```python
from build123d import *

# Parameters (mm, degrees)
SALIENTE_EXTRUIR1_DEPTH = 25.2


with BuildPart() as part:
    # Croquis1 → Saliente-Extruir1 (new body)
    with BuildSketch(Plane(origin=(0, 0, 0), x_dir=(1, 0, 0), z_dir=(0, 1, 0))):
        with BuildLine():
            Line((-2.5, 11.55), (2.5, 11.55))
            Line((2.5, 11.55), (2.5, 9.16515139))
            ThreePointArc((2.5, 9.16515139), (0, -9.5), (-2.5, 9.16515139))
            Line((-2.5, 9.16515139), (-2.5, 11.55))
        make_face()
        with BuildLine():
            Line((-2.439487651, 3.17), (2.439487651, 3.17))
            ThreePointArc((2.439487651, 3.17), (0, -4), (-2.439487651, 3.17))
        make_face(mode=Mode.SUBTRACT)
    extrude(amount=SALIENTE_EXTRUIR1_DEPTH)


solid = part.part
```
Check sheet for the modelled part. Datum: model origin and axes. Units: mm. A direction names the side the tool comes from. Give positions to 0.01 mm unless a question says otherwise; leave off trailing zeros. Order: outer loops, then holes, each group sorted by start corner. A loop starts at its lowest first (then second) coordinate and runs counter-clockwise, first axis right, second up. Notation, with made-up numbers: (43, 49.5) -> (90, 49.5) arc R15 ccw to (90, 65.5) -> close; hole circle Ø3 at (-13.5, 63). An arc over 180 degrees is marked (long way). Return JSON: item names as keys, results as strings.
1. Cross-section at A-A, the plane x = 0. Record the cut outline in (y, z).
From the geometry:
{"outline": "(0, -11.55) -> (25.2, -11.55) -> (25.2, -3.17) -> (0, -3.17) -> close; (0, 4) -> (25.2, 4) -> (25.2, 9.5) -> (0, 9.5) -> close"}
2. Mould release check, pull along X, two halves, no side actions. Record for faces 4 (the flat face through (2.5, 12, -10)), 5 (the cylindrical face through (0, 12, 4)), 6 (the cylindrical face through (0.382, 12.424, 9.492)): +X half, -X half, draft (parallel to the pull), parting line (faces both ways), or undercut.
From the geometry:
{"face 4": "+X half", "face 5": "undercut", "face 6": "parting line"}
3. Cross-section at C-C, the plane y = 13.75. Record the cut outline in (x, z).
From the geometry:
{"outline": "(-2.5, -11.55) -> (2.5, -11.55) -> (2.5, -9.17) arc R9.5 ccw (long way) to (-2.5, -9.17) -> close; hole (-2.44, -3.17) -> (2.44, -3.17) arc R4 ccw (long way) to start"}
4. Set-up check for faces 1 (the flat face through (0, 12, -3.17)), 2 (the flat face through (-2.5, 12, -10)), 3 (the flat face through (0, 12, -11.55)): record each of +Z, -Z, +X, -X, +Y, -Y from which the full face is reachable in a straight line by a thin tool's end or side.
From the geometry:
{"face 1": "+Y, -Y", "face 2": "-Z, -X, +Y, -Y", "face 3": "-Z, +X, -X, +Y, -Y"}
5. Material ranges on probe 1 along X at (y, z) = (12, 0); probe 2 along Z at (x, y) = (0.25, 9.25); probe 3 along Z at (x, y) = (-1.25, 5.75), recorded low to high. Write a range as [from, to].
From the geometry:
{"probe 1": "[-9.5, -4], [4, 9.5]", "probe 2": "[-11.55, -3.17], [3.99, 9.5]", "probe 3": "[-11.55, -3.17], [3.8, 9.42]"}
6. Cross-section at D-D, the plane z = 5.5. Record the cut outline in (x, y), plus the area to 3 significant figures.
From the geometry:
{"outline": "(-7.75, 0) -> (7.75, 0) -> (7.75, 25.2) -> (-7.75, 25.2) -> close", "area": "390 mm^2"}
7. Go/stop test with flat-tipped pins: P1, Ø1, axis at y = 5, z = 5, coming from the -X side; P2, Ø10, axis at y = 20, z = 7, coming from the +X side; P3, Ø4, axis at y = 6.5, z = -6.5, coming from the +X side. Record where each tip stops, or that it passes through.
From the geometry:
{"P1": "x = -8.37", "P2": "x = 9.29", "P3": "x = 8.37"}
8. Cross-section at B-B, the plane z = 0. Record the cut outline in (x, y), plus the area to 3 significant figures.
From the geometry:
{"outline": "(-9.5, 0) -> (-4, 0) -> (-4, 25.2) -> (-9.5, 25.2) -> close; (4, 0) -> (9.5, 0) -> (9.5, 25.2) -> (4, 25.2) -> close", "area": "277 mm^2"}
